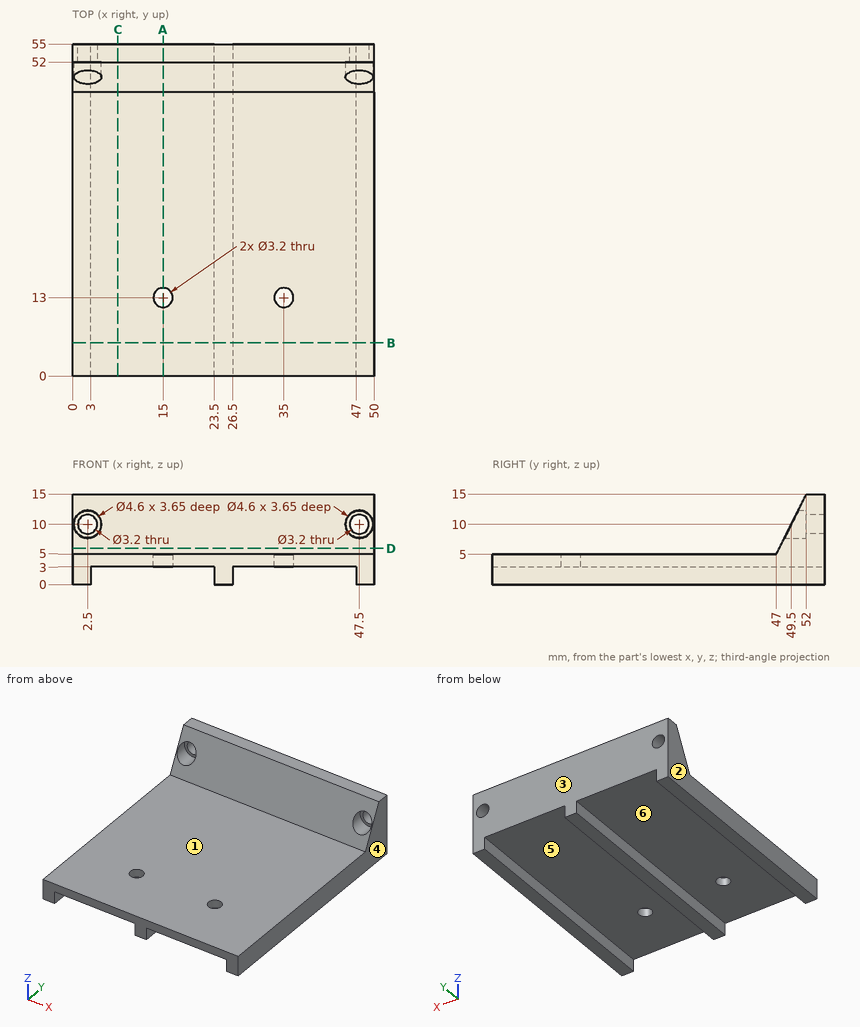
The drawing under review shows one solid part. Ordinate dimensions are in mm from its lowest x, y, z. A direction names the side the tool comes from. Round coordinates to 2 decimals unless told otherwise and drop trailing zeros. Loops run counter-clockwise (first coordinate to the right, second up) from the corner with the lowest first, then second, coordinate; pieces in that order, holes last. Notation, with made-up numbers: (69.25, 34.5) -> (125.25, 34.5) arc R20 ccw to (125.25, 73.5) -> close; hole circle Ø9 at (42, 13.25). An arc over 180 degrees is marked (long way). Answer in a Markdown table with one row per item.
1) Wall thickness on line 1 along X through (y, z) = (19.5, 2); line 2 along Z through (x, y) = (2.5, 49.25); line 3 along Z through (x, y) = (11.5, 23): over which ranges is each line inside the solid? List them lowest first.
Taken from the geometry:
| item | result |
|---|---|
| line 1 | x = 0 to 3, 23.5 to 26.5, 47 to 50 |
| line 2 | z = 0 to 7.7 |
| line 3 | z = 3 to 5 |
2) For pin 1 Ø3.5 at (x, z) = (47.5, 10) entering from -Y; pin 2 Ø14 at (x, y) = (15, 20.5) entering from +Z; pin 3 Ø4 at (x, z) = (2.5, 10) entering from +Y; pin 4 Ø5 at (x, y) = (15, 13) entering from -Z, all flat-tipped, find the tip position at first contact; note any pin that passes through.
Taken from the geometry:
| item | result |
|---|---|
| pin 1 | stops at y = 52 |
| pin 2 | stops at z = 5 |
| pin 3 | stops at y = 55 |
| pin 4 | stops at z = 3 |
3) Draft analysis for pull direction X (two halves, no side actions). For the marked faces 3, 4, 5 and 6, state which applies: pulls with the +X half, pulls with the -X half, needs draft (parallel to the pull), parting line crosses it, or undercut.
Taken from the geometry:
| item | result |
|---|---|
| face 3 | needs draft |
| face 4 | pulls with the +X half |
| face 5 | undercut |
| face 6 | undercut |
4) Consider section D-D, the plane z = 6. Write out the cut boundary in (x, y), plus the area to 3 significant figures.
Taken from the geometry:
| item | result |
|---|---|
| outline | (0, 47.5) -> (50, 47.5) -> (50, 55) -> (0, 55) -> close |
| area | 375 mm² |
5) Consider section C-C, the plane x = 7.5. Write out the cut boundary in (y, z), plus the area to 3 significant figures.
Taken from the geometry:
| item | result |
|---|---|
| outline | (0, 3) -> (55, 3) -> (55, 15) -> (52, 15) -> (47, 5) -> (0, 5) -> close |
| area | 165 mm² |
6) Consider section B-B, the plane y = 5.5. Write out the cut boundary in (x, z), plus the area to 3 significant figures.
Taken from the geometry:
| item | result |
|---|---|
| outline | (0, 0) -> (3, 0) -> (3, 3) -> (23.5, 3) -> (23.5, 0) -> (26.5, 0) -> (26.5, 3) -> (47, 3) -> (47, 0) -> (50, 0) -> (50, 5) -> (0, 5) -> close |
| area | 127 mm² |
7) Tool access review of the marked faces 1 and 2: name each direction out of +Z, -Z, +X, -X, +Y, -Y from which nothing blocks a thin tool from reaching the whole face with its end or side.
Taken from the geometry:
| item | result |
|---|---|
| face 1 | +Z, +X, -X, -Y |
| face 2 | +Z, -Z, -X, +Y, -Y |
8) Consider section A-A, the plane x = 15. Write out the cut boundary in (y, z).
Taken from the geometry:
| item | result |
|---|---|
| outline | (0, 3) -> (11.4, 3) -> (11.4, 5) -> (0, 5) -> close; (14.6, 3) -> (55, 3) -> (55, 15) -> (52, 15) -> (47, 5) -> (14.6, 5) -> close |
